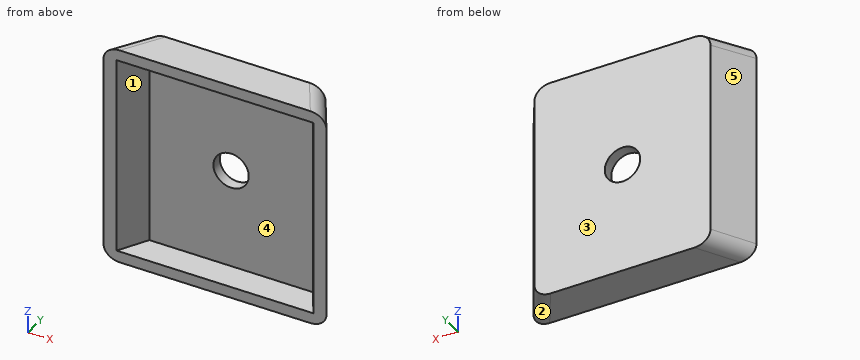
Autodesk Fusion 360 part; units mm, degrees
sketch "bottom" plane through (0, 0, 0) normal (0, 1, 0) x (1, 0, 0)
  line L0 (0, 0) -> (40, 0)
  line L1 (40, 0) -> (40, 39.5)
  line L2 (40, 39.5) -> (0, 39.5)
  line L3 (0, 39.5) -> (0, 0)
  dimension "d4" = 40
  dimension "d5" = 39.5
extrude "Extrude1" add sketch "bottom" along normal blind 7
draft "Draft1" angle 1 neutral plane through (0, 0, 0) pull (0, 1, 0) 1 faces at (13.3333, 2.3333, 0)
draft "Draft2" angle 31 neutral plane through (0, 0, 0) pull (0, 1, 0) 2 faces at (0, 2.3333, -13.2074) (40, 2.3333, -13.2074)
draft "Draft3" angle 1 neutral plane through (0, 0, 0) pull (0, 1, 0) 1 faces at (14.7353, 2.3333, -39.5)
shell "Shell1" thickness 2 removed faces 1 at (26.6667, 0, -13.1667)
sketch "top" plane through (0, 7, 0) normal (0, 1, 0) x (-1, 0, 0)
  line L0 (-4.206, -39.3778) -> (-4.206, -0.1222)
  line L1 (-4.206, -0.1222) -> (-35.794, -0.1222)
  line L2 (-35.794, -0.1222) -> (-35.794, -39.3778)
  line L3 (-35.794, -39.3778) -> (-4.206, -39.3778)
  line L4 (-20, -0.1222) -> (-20, -19.6222) construction
  circle A0 centre (-20, -19.6222) radius 3.175
  dimension "d23" = 19.5
  dimension "d25" = 6.35
extrude "Extrude2" cut sketch "top" against normal blind 2 contours A0
fillet "Fillet1" radius 2.5 4 edges at (2.103, 3.5, -0.0611) (37.897, 3.5, -0.0611) (37.897, 3.5, -39.4389) (2.103, 3.5, -39.4389)
sketch "Sketch3" plane through (0, 0, 0) normal (0, 0.0175, 0.9998) x (1, 0, 0)
  line L0 (37.1096, 0) -> (32.9036, 7.0011)
  line L1 (32.9036, 7.0011) -> (7.0964, 7.0011)
  line L2 (7.0964, 7.0011) -> (2.8904, 0)
  line L3 (2.8904, 0) -> (37.1096, 0)
  line L4 (20, 7.0011) -> (20, 0) construction
  line L5 (4.9934, 3.5005) -> (35.0066, 3.5005) construction
  line L6 (4.9934, 1.7505) -> (35.0066, 1.7505) construction
  dimension "d31" = 1.75
  dimension "d32" = 3.5
extrude "Extrude3" [suppressed]
equation "PLATE_BASE_WIDTH = 40 mm"
equation "PLATE_BASE_HEIGHT = 39.5 mm"
equation "PLATE_HEIGHT = 7 mm"
equation "d4 = PLATE_BASE_WIDTH"
equation "d5 = PLATE_BASE_HEIGHT"
equation "d6 = PLATE_HEIGHT"
equation "DRAFT_SIDES = 31 deg"
equation "DRAFT_BACK = 1 deg"
equation "DRAFT_FRONT = 1 deg"
equation "d14 = DRAFT_FRONT"
equation "d16 = DRAFT_SIDES"
equation "d17 = DRAFT_SIDES"
equation "d18 = DRAFT_BACK"
equation "SHELL_THICKNESS = 2 mm"
equation "d21 = SHELL_THICKNESS"
equation "THREAD_OFFSET_FRONT = 20 mm"
equation "d23 = PLATE_BASE_HEIGHT - THREAD_OFFSET_FRONT"
equation "THREAD_HOLE_RAD = 0.25 in"
equation "d25 = THREAD_HOLE_RAD"
equation "EDGE_FILLET = 2.5 mm"
equation "d30 = EDGE_FILLET"
equation "d31 = PLATE_HEIGHT / 4"
equation "d32 = PLATE_HEIGHT / 2"
For this review, take the finished solid that the model builds, in its own axes (mm). Face numbers are marked on the shaded views. A direction names the side the tool comes from. Round coordinates to 2 decimals unless told otherwise and drop trailing zeros. Order: outer loops, then holes, each group sorted by start corner. A loop starts at its lowest first (then second) coordinate and runs counter-clockwise, first axis right, second up. Notation, with made-up numbers: (44.5, 20) -> (78.5, 20) arc R19 ccw to (78.5, 30) -> close; hole circle Ø8 at (-23.5, 5). An arc over 180 degrees is marked (long way). Write item = value, one per line. Start each with the question number.
1) Take a section at A-A on z = -6. State the section outline as (x, y) points.
2) Tool access review of the marked faces 1 and 2: name each direction out of +Z, -Z, +X, -X, +Y, -Y from which nothing blocks a thin tool from reaching the whole face with its end or side.
3) The part is to be moulded in two halves that separate along X. For the marked faces 3, 4 and 5, say which applies: +X half, -X half, draft (parallel to the pull), parting line (faces both ways), or undercut.
4) Take a section at B-B on x = 20. State the section outline as (y, z) points.
5) To check wall thickness, follow line 1 (Z direction, x = 20, y = 6.3); line 2 (Y direction, x = 16, z = -13); line 3 (X direction, y = 1.5, z = -3). State the ranges of each line that lie inside material, in increasing order. Write a range as from..to.
6) Insertion check: pin 1 (10 mm diameter, centred on x = 5.5, z = -22.5, fed in from -Y); pin 2 (3 mm diameter, centred on x = 34.5, z = -11, fed in from -Y); pin 3 (4 mm diameter, centred on y = 5, z = -10.5, fed in from -X); pin 4 (12 mm diameter, centred on x = 19, z = -10.5, fed in from -Y). Each pin has a flat end and moves straight along its axis. Give the tip position at first contact, or say it passes through.
Verdict:
q1.outline = (0, 0) -> (2.33, 0) -> (5.34, 5) -> (34.66, 5) -> (37.67, 0) -> (40, 0) -> (35.79, 7) -> (4.21, 7) -> close
q2.face_1 = -Y
q2.face_2 = -Z, +X, +Y
q3.face_3 = draft
q3.face_4 = undercut
q3.face_5 = -X half
q4.outline = (0, -39.5) -> (7, -39.38) -> (7, -22.8) -> (5, -22.8) -> (5, -37.41) -> (0, -37.5) -> close; (0, -2) -> (5, -2.09) -> (5, -16.45) -> (7, -16.45) -> (7, -0.12) -> (0, 0) -> close
q5.line_1 = -39.39..-22.8, -16.45..-0.11
q5.line_2 = 5..7
q5.line_3 = 0.9..3.23, 36.77..39.1
q6.pin_1 = 0
q6.pin_2 = 2.77
q6.pin_3 = 1.8
q6.pin_4 = 5
